from build123d import *

# Parameters (mm, degrees)
F0_W     = 63.8048
F0_H     = 15.8242
F1_DEPTH = 9.6139
F2_R     = 2.44475
F3_DEPTH = 1.8415
F4_W     = 62.031426
F4_H     = 13.85646
F5_DEPTH = 8.382
F6_R     = 3.4163
F7_DEPTH = 8.382
F8_R     = 2.54
F9_DEPTH = 8.382


with BuildPart() as f1:
    # F0 (on Top) → F1 (new body)
    with BuildSketch(Plane.XY):
        Rectangle(F0_W, F0_H)
    extrude(amount=F1_DEPTH)

    # F2 (on face) → F3 (join)
    with BuildSketch(Plane.XY.offset(9.6139)):
        with Locations((-27.76855, 3.77825)):
            Circle(F2_R)
        with Locations((11.58875, -3.77825)):
            Circle(F2_R)
        with Locations((-3.49885, -3.77825)):
            Circle(F2_R)
        with Locations((3.49885, -3.77825)):
            Circle(F2_R)
        with Locations((19.67865, -3.77825)):
            Circle(F2_R)
        with Locations((27.76855, -3.77825)):
            Circle(F2_R)
        with Locations((27.76855, 3.77825)):
            Circle(F2_R)
        with Locations((19.67865, 3.77825)):
            Circle(F2_R)
        with Locations((11.58875, 3.77825)):
            Circle(F2_R)
        with Locations((-27.76855, -3.77825)):
            Circle(F2_R)
        with Locations((3.49885, 3.77825)):
            Circle(F2_R)
        with Locations((-3.49885, 3.77825)):
            Circle(F2_R)
        with Locations((-11.58875, 3.77825)):
            Circle(F2_R)
        with Locations((-11.58875, -3.77825)):
            Circle(F2_R)
        with Locations((-19.67865, -3.77825)):
            Circle(F2_R)
        with Locations((-19.67865, 3.77825)):
            Circle(F2_R)
    extrude(amount=F3_DEPTH)

    # F4 (on face) → F5 (cut)
    with BuildSketch(Plane(origin=(0, 0, 0), x_dir=(1, 0, 0), z_dir=(0, 0, -1))):
        Rectangle(F4_W, F4_H)
    extrude(amount=-F5_DEPTH, mode=Mode.SUBTRACT)

    # F6 (on face) → F7 (join)
    with BuildSketch(Plane(origin=(0, 0, 8.382), x_dir=(1, 0, 0), z_dir=(0, 0, -1))):
        with Locations((-16.245613, 0)):
            Circle(F6_R)
        with Locations((-24.399013, 0)):
            Circle(F6_R)
        Circle(F6_R)
        with Locations((-8.092213, 0)):
            Circle(F6_R)
        with Locations((8.092213, 0)):
            Circle(F6_R)
        with Locations((24.399013, 0)):
            Circle(F6_R)
        with Locations((16.245613, 0)):
            Circle(F6_R)
    extrude(amount=F7_DEPTH)

    # F8 (on face) → F9 (cut)
    with BuildSketch(Plane(origin=(0, 0, 0), x_dir=(1, 0, 0), z_dir=(0, 0, -1))):
        with Locations((-24.399013, 0)):
            Circle(F8_R)
        with Locations((-16.245613, 0)):
            Circle(F8_R)
        with Locations((-8.092213, 0)):
            Circle(F8_R)
        Circle(F8_R)
        with Locations((8.092213, 0)):
            Circle(F8_R)
        with Locations((16.245613, 0)):
            Circle(F8_R)
        with Locations((24.399013, 0)):
            Circle(F8_R)
    extrude(amount=-F9_DEPTH, mode=Mode.SUBTRACT)


solid = f1.part
Geometry: final body of the model. Coordinates: model frame, mm. A direction names the side the tool comes from. Give positions to 0.01 mm unless a question says otherwise; leave off trailing zeros. Write each loop counter-clockwise with the first axis right and the second up, starting at its lowest first coordinate (ties: lowest second). Pieces come first, ordered by that corner, then holes. Notation, with made-up numbers: (75, 81) - (117, 81) arc R7 ccw to (117, 87) - close; hole circle Ø6 at (-26.5, -5.75). An arc over 180 degrees is marked (long way). Return JSON: item names as keys, results as strings. Group by question number.
1) Mould query, pull axis X, two halves, no side actions, for faces 4 (the flat face through (-24, -3, 0)), 5 (the cylindrical face through (-17.35, -3.04, 10.52)). Classes: released by +X, released by -X, zero draft, split by the parting line, or undercut.
2) Section A-A on z = 7.25. State how many separate pieces and enclosed holes the cut face has, plus the area to 3 significant figures.
3) First-contact query: P1, Ø2.5, axis at x = -1, y = -0.5, coming from the -Z side; P2, Ø2, axis at x = 17, y = 4, coming from the -Z side; P3, Ø2, axis at x = -7, y = 3.5, coming from the +Z side. Flat tips, straight axial feed; report the tip coordinate or a pass-through.
4) Section C-C on x = -24.5. Return the cut outline in (y, z).
5) Section B-B on x = 0. Return the cut outline in (y, z), plus the area to 3 significant figures.
6) Set-up query: faces 1 (the cylindrical face through (1.56, -5.27, 10.52)), 2 (the flat face through (-20, 4, 11.455)), 3 (the flat face through (-16, 0, 8.382)). Return all of +Z, -Z, +X, -X, +Y, -Y with unobstructed straight access to the full face (end or side cutting, diameter ignored); none if empty.
7) Line query: line 1 (Y direction, x = 0, z = 2); line 2 (Y direction, x = 12, z = 1.5); line 3 (X direction, y = 4.75, z = 7.75). Output: solid intervals per line, ascending.
Filled in:
{
 "1": {"face 4": "zero draft", "face 5": "undercut"},
 "2": {"separate pieces": "8", "enclosed holes": "8", "area": "265 mm^2"},
 "3": {"P1": "stops at z = 8.38", "P2": "stops at z = 0", "P3": "stops at z = 9.61"},
 "4": {"outline": "(-7.91, 0) - (-6.93, 0) - (-6.93, 8.38) - (-3.41, 8.38) - (-3.41, 0) - (-2.54, 0) - (-2.54, 8.38) - (2.54, 8.38) - (2.54, 0) - (3.41, 0) - (3.41, 8.38) - (6.93, 8.38) - (6.93, 0) - (7.91, 0) - (7.91, 9.61) - (-7.91, 9.61) - close"},
 "5": {"outline": "(-7.91, 0) - (-6.93, 0) - (-6.93, 8.38) - (-3.42, 8.38) - (-3.42, 0) - (-2.54, 0) - (-2.54, 8.38) - (2.54, 8.38) - (2.54, 0) - (3.42, 0) - (3.42, 8.38) - (6.93, 8.38) - (6.93, 0) - (7.91, 0) - (7.91, 9.61) - (-7.91, 9.61) - close", "area": "50.7 mm^2"},
 "6": {"face 1": "+Z", "face 2": "+Z, +X, -X, +Y, -Y", "face 3": "-Z"},
 "7": {"line 1": "y = -7.91 to -6.93, -3.42 to -2.54, 2.54 to 3.42, 6.93 to 7.91", "line 2": "y = -7.91 to -6.93, 6.93 to 7.91", "line 3": "x = -31.9 to -31.02, 31.02 to 31.9"}
}
